For this review, use the dimensioned drawing (mm, ordinates from the lowest corner) and the shaded views. A direction names the side the tool comes from. Round coordinates to 2 decimals unless told otherwise and drop trailing zeros. Loops run counter-clockwise (first coordinate to the right, second up) from the corner with the lowest first, then second, coordinate; pieces in that order, holes last. Notation, with made-up numbers: (44, 38.25) - (66, 38.25) arc R16 ccw to (66, 65.25) - close; hole circle Ø9 at (50.5, 30). An arc over 180 degrees is marked (long way). Answer as CSV lines item,"result". Start each with the question number.
(1) Wall thickness on L1, parallel to Z at x = 110, y = 5.1; L2, parallel to Z at x = 110, y = 2.4; L3, parallel to X at y = 0.8, z = 10: over which ranges is each line inside the solid? List them lowest first.
(2) Consider section C-C (z = 10). Give the boundary of the cut face in (x, y), and give its area (3 significant figures).
(3) Consider section D-D (z = 50). Give the boundary of the cut face in (x, y).
(4) Consider section B-B (x = 110). Give the boundary of the cut face in (y, z), and give its area (3 significant figures).
(5) For the marked faces 1 and 2, list the 3-axis set-ups (+Z, -Z, +X, -X, +Y, -Y) from which the entire face can be reached by the end or side of a thin tool; tool diameter is ignored.
(6) For P1, Ø12, axis at x = 110, z = 90, coming from the +Y side; P2, Ø1.5, axis at y = 9, z = 52, coming from the +X side; P3, Ø3.5, axis at x = 8, z = 10, coming from the +Y side, all flat-tipped, find the tip position at first contact; note any pin that passes through.
(7) Consider section A-A (y = 2). Give the boundary of the cut face in (x, z).
(8) Mouldability with a two-part tool opening along Z and no side actions: class the marked faces 3 and 4 as released by +Z, released by -Z, zero draft, split by the parting line, or undercut.
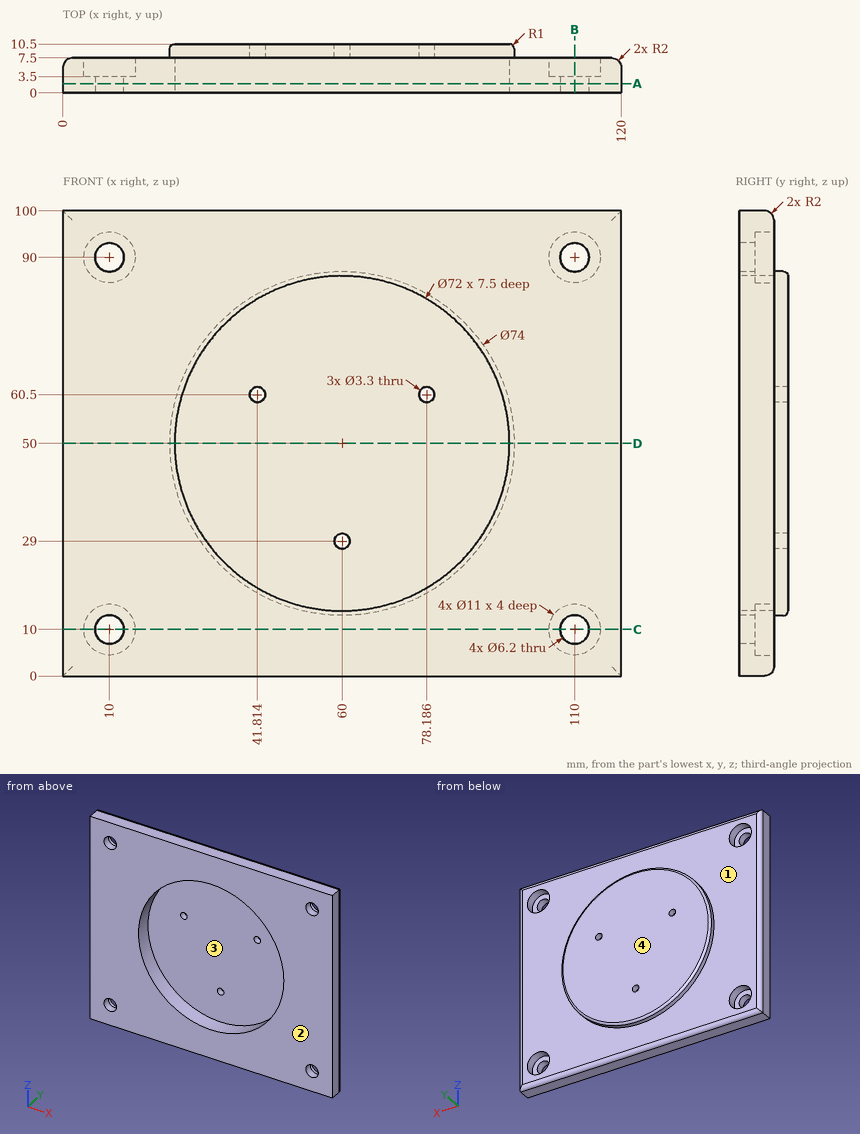
Determined:
1,L1,"z = 0 to 4.5, 15.5 to 84.5, 95.5 to 100"
1,L2,"z = 0 to 6.9, 13.1 to 86.9, 93.1 to 100"
1,L3,"x = 0 to 6.9, 13.1 to 106.9, 113.1 to 120"
2,outline,"(0, 0) - (6.9, 0) - (6.9, 3.5) - (4.5, 3.5) - (4.5, 7.5) - (2, 7.5) arc R2 ccw to (0, 5.5) - close; (13.1, 0) - (106.9, 0) - (106.9, 3.5) - (104.5, 3.5) - (104.5, 7.5) - (15.5, 7.5) - (15.5, 3.5) - (13.1, 3.5) - close; (113.1, 0) - (120, 0) - (120, 5.5) arc R2 ccw to (118, 7.5) - (115.5, 7.5) - (115.5, 3.5) - (113.1, 3.5) - close"
2,area,"767 mm^2"
3,outline,"(0, 0) - (24, 0) - (24, 7.5) - (96, 7.5) - (96, 0) - (120, 0) - (120, 5.5) arc R2 ccw to (118, 7.5) - (97, 7.5) - (97, 9.5) arc R1 ccw to (96, 10.5) - (24, 10.5) arc R1 ccw to (23, 9.5) - (23, 7.5) - (2, 7.5) arc R2 ccw to (0, 5.5) - close"
4,outline,"(0, 0) - (5.5, 0) arc R2 ccw to (7.5, 2) - (7.5, 4.5) - (3.5, 4.5) - (3.5, 6.9) - (0, 6.9) - close; (0, 13.1) - (3.5, 13.1) - (3.5, 15.5) - (7.5, 15.5) - (7.5, 84.5) - (3.5, 84.5) - (3.5, 86.9) - (0, 86.9) - close; (0, 93.1) - (3.5, 93.1) - (3.5, 95.5) - (7.5, 95.5) - (7.5, 98) arc R2 ccw to (5.5, 100) - (0, 100) - close"
4,area,"617 mm^2"
5,face 1,"+Y"
5,face 2,"+Z, -Z, +X, -X, -Y"
6,P1,"stops at y = 7.5"
6,P2,"stops at x = 96.98"
6,P3,"stops at y = 3.5"
7,outline,"(0, 0) - (120, 0) - (120, 100) - (0, 100) - close; hole circle Ø6.2 at (10, 10); hole circle Ø6.2 at (10, 90); hole circle Ø72 at (60, 50); hole circle Ø6.2 at (110, 10); hole circle Ø6.2 at (110, 90)"
8,face 3,"undercut"
8,face 4,"zero draft"
